Source: CAD feature listing. Evaluate the final solid. Frame: model axes, mm. Face numbers are marked on the shaded views. Give positions to 0.01 mm unless a question says otherwise; leave off trailing zeros. Order: outer loops, then holes, each group sorted by start corner. A loop starts at its lowest first (then second) coordinate and runs counter-clockwise, first axis right, second up.
1) Section B-B, the plane y = -11. Return loops of the section in (x, z), plus the area to 3 significant figures.
2) Material intervals for line 1 (X direction, y = 21, z = 1.1); line 2 (Y direction, x = -33.5, z = 0.95); line 3 (Z direction, x = 36, y = -19.5), sorted ascending.
3) Section D-D, the plane x = 24. Return loops of the section in (y, z), plus the area to 3 significant figures.
4) Section C-C, the plane z = 0.55. Return loops of the section in (x, y).
5) Section A-A, the plane x = 13. Return loops of the section in (y, z).
6) Draft query along X for the marked faces 1 and 2. Return one class per face: released by +X, released by -X, zero draft, split by the parting line, or undercut.
```python
from build123d import *

# Parameters (mm, degrees)
SKETCH1_W           = 98.5
SKETCH1_H           = 80.4
SKETCH1_W_2         = 90.6
SKETCH1_H_2         = 68.2
BOSS_EXTRUDE1_DEPTH = 1.2
SKETCH1_3_W         = 90.6
SKETCH1_3_H         = 68.2
BOSS_EXTRUDE2_DEPTH = 0.9
SKETCH1_4_W         = 25.5
SKETCH1_4_H         = 8
BOSS_EXTRUDE3_DEPTH = 0.3


with BuildPart() as part:
    # Sketch1 → Boss-Extrude1 (new body)
    with BuildSketch(Plane.XY):
        with Locations((0.65, 2.8)):
            Rectangle(SKETCH1_W, SKETCH1_H)
        Rectangle(SKETCH1_W_2, SKETCH1_H_2, mode=Mode.SUBTRACT)
    extrude(amount=BOSS_EXTRUDE1_DEPTH)

    # Sketch1_3 → Boss-Extrude2 (add)
    with BuildSketch(Plane.XY):
        Rectangle(SKETCH1_3_W, SKETCH1_3_H)
    extrude(amount=BOSS_EXTRUDE2_DEPTH)

    # Sketch1_4 → Boss-Extrude3 (add)
    with BuildSketch(Plane.XY):
        with Locations((6.05, 47)):
            Rectangle(SKETCH1_4_W, SKETCH1_4_H)
    extrude(amount=BOSS_EXTRUDE3_DEPTH)


solid = part.part
```
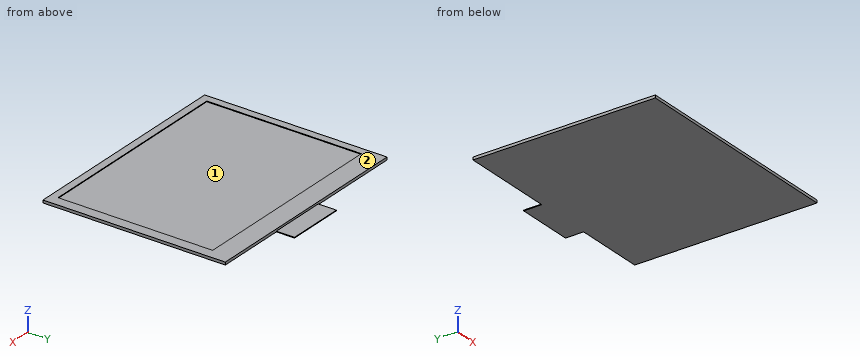
From the geometry:
1. outline: (-48.6, 0) - (49.9, 0) - (49.9, 1.2) - (45.3, 1.2) - (45.3, 0.9) - (-45.3, 0.9) - (-45.3, 1.2) - (-48.6, 1.2) - close
1. area: 91.0 mm2
2. line 1: x = -48.6 to -45.3, 45.3 to 49.9
2. line 2: y = -37.4 to -34.1, 34.1 to 43
2. line 3: z = 0 to 0.9
3. outline: (-37.4, 0) - (43, 0) - (43, 1.2) - (34.1, 1.2) - (34.1, 0.9) - (-34.1, 0.9) - (-34.1, 1.2) - (-37.4, 1.2) - close
3. area: 76.0 mm2
4. outline: (-48.6, -37.4) - (49.9, -37.4) - (49.9, 43) - (-48.6, 43) - close
5. outline: (-37.4, 0) - (51, 0) - (51, 0.3) - (43, 0.3) - (43, 1.2) - (34.1, 1.2) - (34.1, 0.9) - (-34.1, 0.9) - (-34.1, 1.2) - (-37.4, 1.2) - close
6. face 1: undercut
6. face 2: zero draft
